```python
from build123d import *

# Parameters (mm, degrees)
EXTRUDE_1_DEPTH         = 3
CUT_EXTRUDE_START       = -3
CUT_EXTRUDE_1_OUTLINE_W = 20
CUT_EXTRUDE_1_OUTLINE_H = 5.5
CUT_EXTRUDE_1_DEPTH     = 3
CUT_EXTRUDE_1_2_DEPTH   = 3


# Read off the part's stored shape, not the designer's step: 切除-拉伸1
with BuildPart() as part:
    # 草图1 → 凸台-拉伸1 (new body)
    with BuildSketch(Plane.XY):
        Polygon((-78.5, 25), (-68.5, 25), (-73.5, 30), (61.5, 30), (56.5, 25), (66.5, 25), (66.5, 10), (61.5, 10), (61.5, 5), (-73.5, 5), (-73.5, 10), (-78.5, 10), align=None)
    extrude(amount=EXTRUDE_1_DEPTH)

    # 切除-拉伸1 outline → 切除-拉伸1 (cut)
    with BuildSketch(Plane.XY.offset(3).offset(CUT_EXTRUDE_START)):
        with Locations((-6, 17.975640355)):
            Rectangle(CUT_EXTRUDE_1_OUTLINE_W, CUT_EXTRUDE_1_OUTLINE_H)
        with Locations((-46, 17.975640355)):
            Rectangle(CUT_EXTRUDE_1_OUTLINE_W, CUT_EXTRUDE_1_OUTLINE_H)
        with Locations((34, 17.975640355)):
            Rectangle(CUT_EXTRUDE_1_OUTLINE_W, CUT_EXTRUDE_1_OUTLINE_H)
    extrude(amount=CUT_EXTRUDE_1_DEPTH, mode=Mode.SUBTRACT)

    # Cut-Extrude 1 2 outline → Cut-Extrude 1 2 (add)
    with BuildSketch(Plane.XY.offset(3).offset(CUT_EXTRUDE_START)):
        Polygon((-78.5, 25), (-80.5, 25), (-80.5, 5), (-75.5, 5), (-75.5, 10), (-78.5, 10), align=None)
        Polygon((68.5, 25), (66.5, 25), (66.5, 10), (63.5, 10), (63.5, 5), (68.5, 5), align=None)
    extrude(amount=CUT_EXTRUDE_1_2_DEPTH)


solid = part.part
```
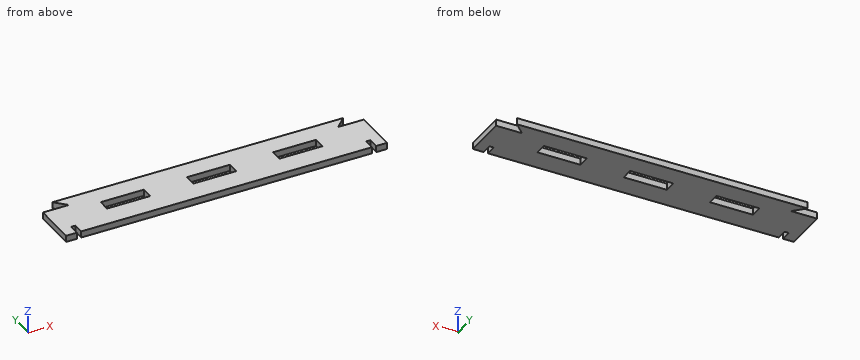
Build history of the part. All positions in model axes, mm. Give positions to 0.01 mm unless a question says otherwise; leave off trailing zeros. Loops run counter-clockwise (first coordinate to the right, second up) from the corner with the lowest first, then second, coordinate; pieces in that order, holes last.
1) Band-saw the part on B-B on x = 36. List the corners of the cut face in (y, z), then the cut area to 3 significant figures.
Values follow:
outline: (5, 0) - (15.23, 0) - (15.23, 3) - (5, 3) - close; (20.73, 0) - (30, 0) - (30, 3) - (20.73, 3) - close
area: 58.5 mm2
2) Band-saw the part on A-A on y = 8. List the corners of the cut face in (x, z), then the cut area to 3 significant figures.
Values follow:
outline: (-80.5, 0) - (-75.5, 0) - (-75.5, 3) - (-80.5, 3) - close; (-73.5, 0) - (61.5, 0) - (61.5, 3) - (-73.5, 3) - close; (63.5, 0) - (68.5, 0) - (68.5, 3) - (63.5, 3) - close
area: 435 mm2
3) Band-saw the part on C-C on z = 0.95. List the corners of the cut face in (x, y), then the cut area to 3 significant figures.
Values follow:
outline: (-80.5, 5) - (-75.5, 5) - (-75.5, 10) - (-73.5, 10) - (-73.5, 5) - (61.5, 5) - (61.5, 10) - (63.5, 10) - (63.5, 5) - (68.5, 5) - (68.5, 25) - (56.5, 25) - (61.5, 30) - (-73.5, 30) - (-68.5, 25) - (-80.5, 25) - close; hole (-56, 15.23) - (-36, 15.23) - (-36, 20.73) - (-56, 20.73) - close; hole (-16, 15.23) - (4, 15.23) - (4, 20.73) - (-16, 20.73) - close; hole (24, 15.23) - (44, 15.23) - (44, 20.73) - (24, 20.73) - close
area: 3,280 mm2
4) Drop a flat-ended pin along its axis: P1, Ø1.6, axis at x = 62.5, z = 2, coming from the -Y side. Give the stop position or say it passes through.
Values follow:
P1: stops at y = 10
5) Probe line 1 along X through (y, z) = (20, 1.45); line 2 along X through (y, z) = (7.25, 0.8); line 3 along Y through (x, z) = (-12, 2.45). List the from-to ranges inside material, lowest first.
Values follow:
line 1: x = -80.5 to -56, -36 to -16, 4 to 24, 44 to 68.5
line 2: x = -80.5 to -75.5, -73.5 to 61.5, 63.5 to 68.5
line 3: y = 5 to 15.23, 20.73 to 30
6) Band-saw the part on D-D on y = 17.75. List the corners of the cut face in (x, z).
Values follow:
outline: (-80.5, 0) - (-56, 0) - (-56, 3) - (-80.5, 3) - close; (-36, 0) - (-16, 0) - (-16, 3) - (-36, 3) - close; (4, 0) - (24, 0) - (24, 3) - (4, 3) - close; (44, 0) - (68.5, 0) - (68.5, 3) - (44, 3) - close
